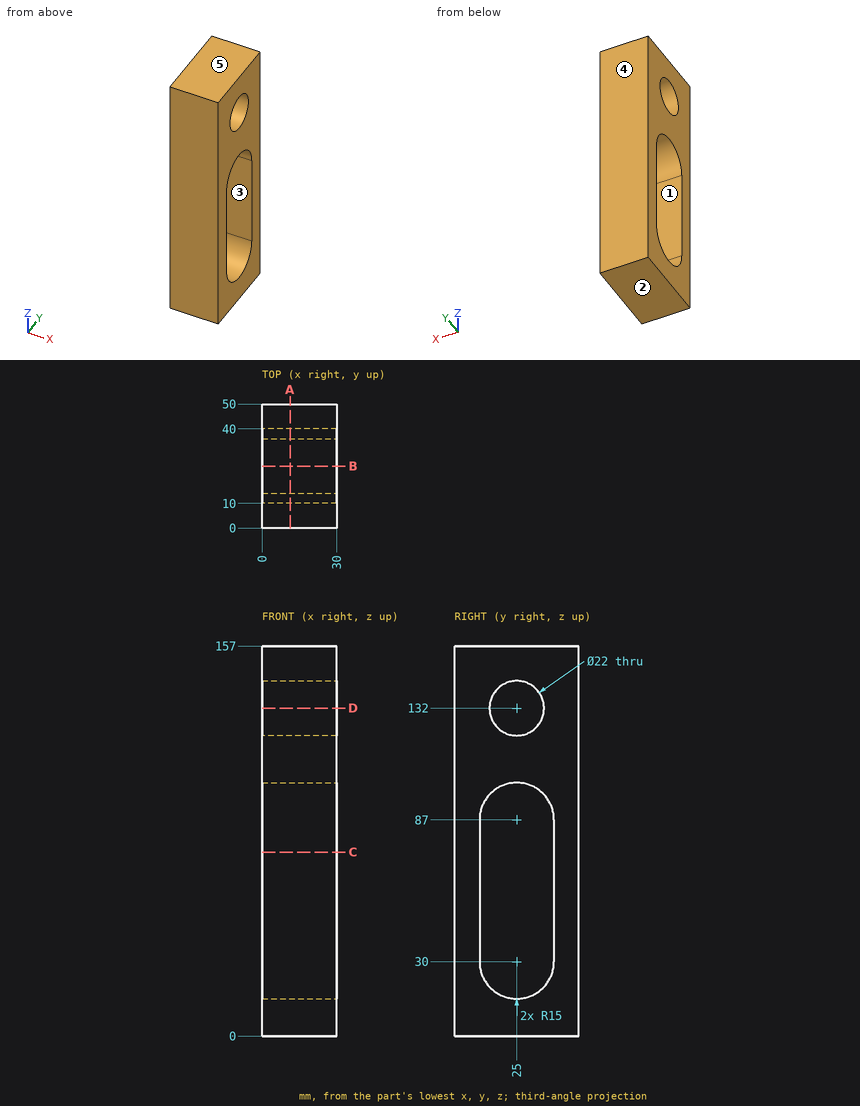
Geometry check sheet. Reference: drawing and pictorial views, mm from the part's lowest x, y, z. A direction names the side the tool comes from. Give positions to 0.01 mm unless a question says otherwise; leave off trailing zeros. Write each loop counter-clockwise with the first axis right and the second up, starting at its lowest first coordinate (ties: lowest second). Pieces come first, ordered by that corner, then holes.
Item 1: Gauge pin test, flat end, axial feed: pin 1 (4 mm diameter, centred on y = 36.5, z = 29.5, fed in from -X). Record the tip position at first contact, or that the pin passes through.
Item 2: Scan lines: L1, parallel to Y at x = 6, z = 49; L2, parallel to Y at x = 7.25, z = 132; L3, parallel to Z at x = 11.5, y = 21. Record each from-to range of solid material in increasing order.
Item 3: Cross-section at A-A (x = 11.25). Enter the section's corners in (y, z).
Item 4: Draft check along Z on the marked faces 3, 4 and 5. Enter one of: released by +Z, released by -Z, zero draft, split by the parting line, or undercut.
Item 5: Access from +Z, -Z, +X, -X, +Y, -Y to the whole of each face (thin tool, end or side, straight path). Record for the marked faces 1 and 2.
Item 6: Cross-section at D-D (z = 132). Enter the section's corners in (x, y).
Item 7: Cross-section at C-C (z = 74). Enter the section's corners in (x, y), and give its area (3 significant figures).
Item 8: Cross-section at B-B (y = 25). Enter the section's corners in (x, z).
Report:
1. pin 1: passes through
2. L1: y = 0 to 10, 40 to 50
2. L2: y = 0 to 14, 36 to 50
2. L3: z = 0 to 15.54, 101.46 to 121.75, 142.25 to 157
3. outline: (0, 0) - (50, 0) - (50, 157) - (0, 157) - close; hole (10, 30) arc R15 ccw to (40, 30) - (40, 87) arc R15 ccw to (10, 87) - close; hole circle Ø22 at (25, 132)
4. face 3: undercut
4. face 4: zero draft
4. face 5: released by +Z
5. face 1: +X, -X
5. face 2: -Z, +X, -X, +Y, -Y
6. outline: (0, 0) - (30, 0) - (30, 14) - (0, 14) - close; (0, 36) - (30, 36) - (30, 50) - (0, 50) - close
7. outline: (0, 0) - (30, 0) - (30, 10) - (0, 10) - close; (0, 40) - (30, 40) - (30, 50) - (0, 50) - close
7. area: 600 mm2
8. outline: (0, 0) - (30, 0) - (30, 15) - (0, 15) - close; (0, 102) - (30, 102) - (30, 121) - (0, 121) - close; (0, 143) - (30, 143) - (30, 157) - (0, 157) - close
